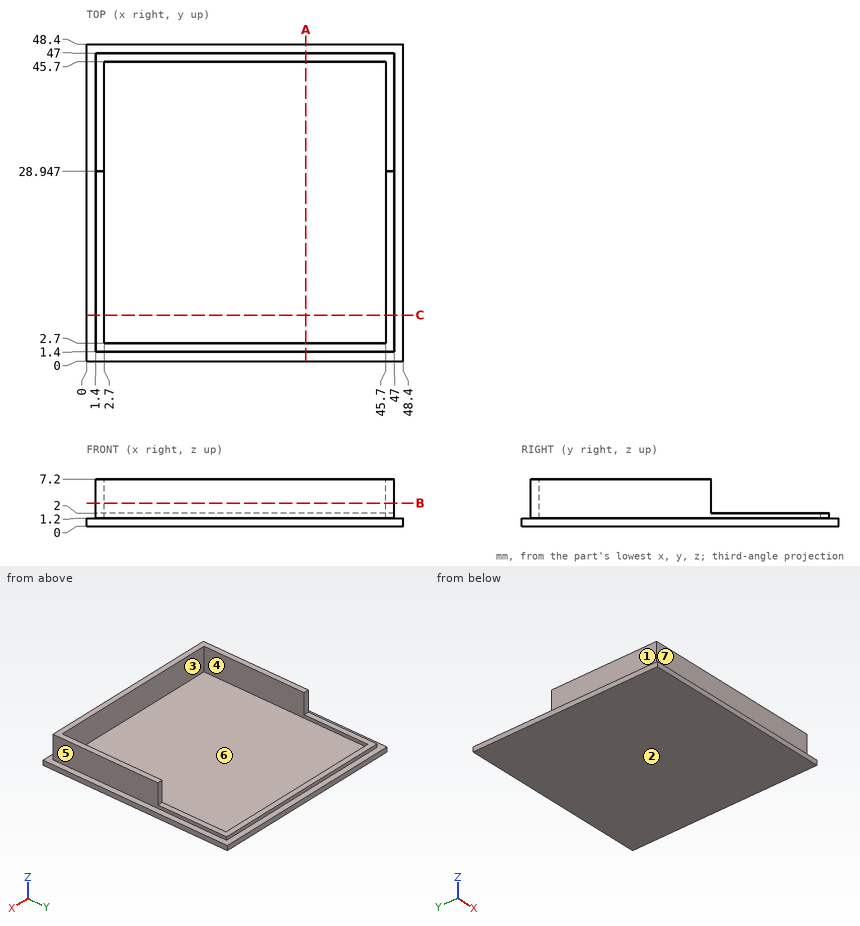
Answer from the drawing. Dimensions are ordinates in mm from the lowest x, y and z of the part. A direction names the side the tool comes from. Coordinates: 2 decimals unless noted, no trailing zeros. Order: outer loops, then holes, each group sorted by start corner. A loop starts at its lowest first (then second) coordinate and runs counter-clockwise, first axis right, second up. Notation, with made-up numbers: (23, 26) - (36, 26) arc R16 ccw to (36, 30) - close; hole circle Ø2 at (39, 62). An arc over 180 degrees is marked (long way). Answer as a JSON object with one key per item and string values. Group by question number.
Item 1: A tool of negligible diameter and unlimited length cuts with its end or side. For the marked faces 5, 6 and 7, from which of +Z, -Z, +X, -X, +Y, -Y can it reach the whole face along a straight path? Write none if from no direction.
Item 2: Section B-B (z = 3.5) is taken. Give the vertices of the cut face in (x, y).
Item 3: Section A-A (x = 33.5) is taken. Give the vertices of the cut face in (y, z).
Item 4: Section C-C (y = 7) is taken. Give the vertices of the cut face in (x, z).
Item 5: Flat-ended cylindrical pins translate along their axes: P1, Ø1.5, axis at y = 27, z = 2.5, coming from the +X side; P2, Ø3, axis at x = 18, z = 4.5, coming from the +Y side; P3, Ø1.4, axis at x = 46.5, z = 5, coming from the +Y side. Find the tip coordinate at first contact, or state that the pin passes through.
Item 6: The mould has two halves that part along X. Classify the marked faces 1, 2, 3 and 4: +X half, -X half, draft (parallel to the pull), parting line (faces both ways), or undercut.
Item 7: Consider probe 1 along Y at (x, z) = (6.5, 1.5); probe 2 along Z at (x, y) = (39.5, 44.5). Determine where each line is inside the solid, lowest interval first. Write a range as from..to.
Results are:
{
 "1": {"face 5": "+Z, +X, +Y, -Y", "face 6": "+Z", "face 7": "+Z, +X, -X, -Y"},
 "2": {"outline": "(1.4, 1.4) - (47, 1.4) - (47, 28.95) - (45.7, 28.95) - (45.7, 2.7) - (2.7, 2.7) - (2.7, 28.95) - (1.4, 28.95) - close"},
 "3": {"outline": "(0, 0) - (48.4, 0) - (48.4, 1.2) - (47, 1.2) - (47, 2) - (45.7, 2) - (45.7, 1.2) - (2.7, 1.2) - (2.7, 7.2) - (1.4, 7.2) - (1.4, 1.2) - (0, 1.2) - close"},
 "4": {"outline": "(0, 0) - (48.4, 0) - (48.4, 1.2) - (47, 1.2) - (47, 7.2) - (45.7, 7.2) - (45.7, 1.2) - (2.7, 1.2) - (2.7, 7.2) - (1.4, 7.2) - (1.4, 1.2) - (0, 1.2) - close"},
 "5": {"P1": "stops at x = 47", "P2": "stops at y = 2.7", "P3": "stops at y = 28.95"},
 "6": {"face 1": "-X half", "face 2": "draft", "face 3": "undercut", "face 4": "undercut"},
 "7": {"probe 1": "y = 1.4..2.7, 45.7..47", "probe 2": "z = 0..1.2"}
}
